Autodesk Inventor part; units mm, degrees
ref_plane "YZ Plane" through (0, 0, 0) normal (1, 0, 0) x (0, 1, 0)
ref_plane "XZ Plane" through (0, 0, 0) normal (0, 1, 0) x (-1, 0, 0)
ref_plane "XY Plane" through (0, 0, 0) normal (0, 0, 1) x (1, 0, 0)
sketch "Sketch1" plane through (0, 0, 0) normal (0, 0, 1) x (1, 0, 0)
  line L0 (0, 0) -> (0, 52)
  line L1 (0, 52) -> (148, 52)
  line L2 (148, 52) -> (148, 0)
  line L3 (148, 0) -> (118, 0)
  line L4 (118, 0) -> (118, 30)
  line L5 (118, 30) -> (30, 30)
  line L6 (30, 30) -> (30, 0)
  line L7 (30, 0) -> (0, 0)
  dimension "d0" = 52
  dimension "d1" = 88
  dimension "d2" = 30
  dimension "d3" = 30
extrude "Extrusion1" add sketch "Sketch1" along normal blind 20
chamfer "Chamfer1" distance 20 angle 45 2 edges at (0, 52, 10) (148, 52, 10)
chamfer "Chamfer4" distance 6 angle 45 2 edges at (118, 30, 10) (30, 30, 10)
sketch "Sketch3" plane through (20, 52, 0) normal (0, 1, 0) x (1, 0, 0)
  line L0 (-20, -20) -> (0, -20)
  line L1 (0, -20) -> (0, 0)
  line L2 (0, 0) -> (-20, 0)
  line L3 (-20, 0) -> (-20, -20)
  line L4 (108, -20) -> (128, -20)
  line L5 (128, -20) -> (128, 0)
  line L6 (128, 0) -> (108, 0)
  line L7 (108, 0) -> (108, -20)
  line L8 (10, 0) -> (-20, 0)
  line L9 (10, 0) -> (10, -20)
  line L10 (-20, -20) -> (10, -20)
  line L11 (-20, 0) -> (-20, -20)
  line L12 (128, 0) -> (98, 0)
  line L13 (128, 0) -> (128, -20)
  line L14 (98, -20) -> (128, -20)
  line L15 (98, 0) -> (98, -20)
  point P0 (-5, -10)
  point P1 (113, -10)
  dimension "d25" = 15
  dimension "d26" = 10
  dimension "d27" = 15
hole "Hole2" at (15, 52, 10) at (133, 52, 10) direction (0, -1, 0) diameter 5.5 end through all counterbore diameter 9 counterbore depth 40
chamfer "Chamfer3" distance 4 angle 45 20 edges at (74, 52, 20) (10, 42, 20) (0, 16, 20) (138, 42, 20) (148, 16, 20) (138, 42, 0) (148, 16, 0) (74, 52, 0) (10, 42, 0) (0, 16, 0) (30, 12, 0) (74, 30, 0) (118, 12, 0) (74, 30, 20) (30, 12, 20) (118, 12, 20) (115, 27, 0) (33, 27, 0) (33, 27, 20) (115, 27, 20)
properties part number "FrameHandle" material "ABS Plastic"
Could you check a few things on this model? Use its own coordinates, in mm. A direction names the side the tool comes from. Give positions to 0.01 mm unless a question says otherwise; leave off trailing zeros. Loops run counter-clockwise (first coordinate to the right, second up) from the corner with the lowest first, then second, coordinate; pieces in that order, holes last. Notation, with made-up numbers: (-38.75, 5.25) -> (-26.75, 5.25) arc R6 ccw to (-26.75, 10.25) -> close; hole circle Ø6 at (54.25, 68). An arc over 180 degrees is marked (long way). Put each result on its own line as item: value.
(1) Thinking about a two-plate mould opening in Z: for faces 1 (the face through (18, 12, 10)), 2 (the face through (30, 12, 10)), 3 (the face through (2, 16, 18)), which applies, pulls with the +Z half, pulls with the -Z half, needs draft (parallel to the pull), parting line crosses it, or undercut?
Computed:
face 1: undercut
face 2: needs draft
face 3: pulls with the +Z half
(2) Imagine slicing it at B-B on z = 10. Write out the boundary of the cut face in (x, y), plus the area to 3 significant figures.
Computed:
outline: (0, 0) -> (12.25, 0) -> (12.25, 12) -> (10.5, 12) -> (10.5, 42.5) -> (0, 32) -> close; (17.75, 0) -> (30, 0) -> (30, 24) -> (36, 30) -> (112, 30) -> (118, 24) -> (118, 0) -> (130.25, 0) -> (130.25, 12) -> (128.5, 12) -> (128.5, 51.5) -> (128, 52) -> (20, 52) -> (19.5, 51.5) -> (19.5, 12) -> (17.75, 12) -> close; (135.75, 0) -> (148, 0) -> (148, 32) -> (137.5, 42.5) -> (137.5, 12) -> (135.75, 12) -> close
area: 3,930 mm^2
(3) Imagine slicing it at A-A on y = 7. Write out the boundary of the cut face in (x, z), plus the area to 3 significant figures.
Computed:
outline: (0, 4) -> (4, 0) -> (26, 0) -> (30, 4) -> (30, 16) -> (26, 20) -> (4, 20) -> (0, 16) -> close; (118, 4) -> (122, 0) -> (144, 0) -> (148, 4) -> (148, 16) -> (144, 20) -> (122, 20) -> (118, 16) -> close; hole circle Ø5.5 at (15, 10); hole circle Ø5.5 at (133, 10)
area: 1,090 mm^2
(4) For faces 4 (the face through (28, 13, 2)), 5 (the face through (115, 27, 10)), 6 (the face through (28, 13, 18)), 7 (the face through (128.54, 31.48, 9.41)), which set-ups out of +Z, -Z, +X, -X, +Y, -Y let a thin tool reach every point of the face, with its end or its side?
Computed:
face 4: -Z, -Y
face 5: +Z, -Z, -Y
face 6: +Z, -Y
face 7: +Y
(5) Imagine slicing it at D-D on x = 98.5. Write out the boundary of the cut face in (y, z).
Computed:
outline: (30, 4) -> (34, 0) -> (48, 0) -> (52, 4) -> (52, 16) -> (48, 20) -> (34, 20) -> (30, 16) -> close
(6) I'm going to push flat-ended pins straight in: pin 1 Ø9.5 at (x, z) = (90.5, 10) entering from -Y; pin 2 Ø4.5 at (x, z) = (14.5, 10.5) entering from +Y; pin 3 Ø6 at (x, z) = (132.5, 14.5) entering from +Y. Where does each tip first touch, or does it pass through?
Computed:
pin 1: y = 30
pin 2: y = 12
pin 3: y = 50.5
(7) Imagine slicing it at C-C on x = 15. Write out the boundary of the cut face in (y, z).
Computed:
outline: (0, 0) -> (41.34, 0) -> (47, 4) -> (47, 5.5) -> (12, 5.5) -> (12, 7.25) -> (0, 7.25) -> close; (0, 12.75) -> (12, 12.75) -> (12, 14.5) -> (47, 14.5) -> (47, 16) -> (41.34, 20) -> (0, 20) -> close
(8) Please list where these lines run through material, in increasing order: probe 1 along X at (y, z) = (9.25, 10); probe 2 along X at (y, z) = (31.5, 10); probe 3 along X at (y, z) = (22, 10.25). Write a range as [from, to].
Computed:
probe 1: [0, 12.25], [17.75, 30], [118, 130.25], [135.75, 148]
probe 2: [0, 10.5], [19.5, 128.5], [137.5, 148]
probe 3: [0, 10.51], [19.49, 30], [118, 128.51], [137.49, 148]
